from build123d import *

# Parameters (mm, degrees)
BOSS_EXTRUDE1_DEPTH = 49
SKETCH2_W           = 306.472298026
SKETCH2_H           = 30.75390082
CUT_EXTRUDE1_DEPTH  = 34
SKETCH4_R           = 3.65
CUT_EXTRUDE2_DEPTH  = 10


with BuildPart() as part:
    # Sketch1 → Boss-Extrude1 (new body)
    with BuildSketch(Plane(origin=(0, 0, 0), x_dir=(0, 0, -1), z_dir=(1, 0, 0))):
        Polygon((-375.84656477, -0.209706312), (-390.875399113, -23.945501074), (-375.84656477, -30.963607132), (-56.374266744, -30.963607132), (-56.374266744, -0.209706312), align=None)
    extrude(amount=BOSS_EXTRUDE1_DEPTH)

    # Sketch2 → Cut-Extrude1 (cut)
    with BuildSketch(Plane.ZY):
        with Locations((214.610415757, -15.586656722)):
            Rectangle(SKETCH2_W, SKETCH2_H)
    extrude(amount=-CUT_EXTRUDE1_DEPTH, mode=Mode.SUBTRACT)

    # Sketch4 → Cut-Extrude2 (cut)
    with BuildSketch(Plane(origin=(0, 0, 56.374266744), x_dir=(-1, 0, 0), z_dir=(0, 0, -1))):
        with Locations((-10, -15.209706312)):
            Circle(SKETCH4_R)
    extrude(amount=-CUT_EXTRUDE2_DEPTH, mode=Mode.SUBTRACT)


solid = part.part
Design review of the part built by this model. Coordinates are the model's own, in mm. A direction names the side the tool comes from. Round coordinates to 2 decimals unless told otherwise and drop trailing zeros. Loops run counter-clockwise (first coordinate to the right, second up) from the corner with the lowest first, then second, coordinate; pieces in that order, holes last. Notation, with made-up numbers: M -17.5,77 L 3.5,77 A31 ccw 3.5,115 Z; hole C 9,46.5 d2. An arc over 180 degrees is marked long. Answer as a JSON object with one key per item and string values.
Item 1: Wall thickness on L1, parallel to Y at x = 10, z = 58; L2, parallel to X at y = -25.5, z = 223.5; L3, parallel to Z at x = 18, y = -1.5: over which ranges is each line inside the solid? List them lowest first. Write a range as from..to.
Answer sheet:
{"L1": "y = -30.96..-18.86, -11.56..-0.21", "L2": "x = 34..49", "L3": "z = 56.37..61.37, 367.85..376.66"}
Item 2: We need section B-B on x = 10. Give the boundary of the cut face in (y, z).
Answer sheet:
{"outline": "M -30.96,56.37 L -18.86,56.37 L -18.86,61.37 L -30.96,61.37 Z; M -30.96,367.85 L -0.21,367.85 L -0.21,375.85 L -23.95,390.88 L -30.96,375.85 Z; M -11.56,56.37 L -0.21,56.37 L -0.21,61.37 L -11.56,61.37 Z"}
Item 3: We need section D-D on z = 148. Give the boundary of the cut face in (x, y).
Answer sheet:
{"outline": "M 34,-30.96 L 49,-30.96 L 49,-0.21 L 34,-0.21 Z"}
Item 4: We need section C-C on x = 43. Give the boundary of the cut face in (y, z), and give its area (3 significant figures).
Answer sheet:
{"outline": "M -30.96,56.37 L -0.21,56.37 L -0.21,375.85 L -23.95,390.88 L -30.96,375.85 Z", "area": "10,100 mm^2"}
Item 5: Machinability: for faces 4 (the flat face through (37, -0.21, 227)), 5 (the flat face through (34, -15, 212)), which of the approach directions +Z, -Z, +X, -X, +Y, -Y give a long, thin tool a straight path to every point of the face, cutting with its end or side? Answer none if there is none.
Answer sheet:
{"face 4": "+Z, -Z, +X, -X, +Y", "face 5": "-X, +Y, -Y"}
Item 6: The part is to be moulded in two halves that separate along Y. For faces 1 (the flat face through (24.157, -27.405, 383.466)), 2 (the cylindrical face through (10.791, -18.773, 58.839)), 3 (the flat face through (17, -16, 367.847)), say which applies: pulls with the +Y half, pulls with the -Y half, needs draft (parallel to the pull), parting line crosses it, or undercut.
Answer sheet:
{"face 1": "pulls with the -Y half", "face 2": "undercut", "face 3": "needs draft"}
Item 7: We need section A-A on x = 31. Give the boundary of the cut face in (y, z).
Answer sheet:
{"outline": "M -30.96,56.37 L -0.21,56.37 L -0.21,61.37 L -30.96,61.37 Z; M -30.96,367.85 L -0.21,367.85 L -0.21,375.85 L -23.95,390.88 L -30.96,375.85 Z"}
Item 8: Clearance check with flat-ended pins moving along their axes: P1, Ø10, axis at x = 33.5, z = 287, coming from the +Y side; P2, Ø10, axis at y = -11, z = 207.5, coming from the -X side. State where each tip first meets the part, or that it passes through.
Answer sheet:
{"P1": "stops at y = -0.21", "P2": "stops at x = 34"}
